Geometry check sheet. Reference: drawing and pictorial views, mm from the part's lowest x, y, z. Give positions to 0.01 mm unless a question says otherwise; leave off trailing zeros. Order: outer loops, then holes, each group sorted by start corner. A loop starts at its lowest first (then second) coordinate and runs counter-clockwise, first axis right, second up. Notation, with made-up numbers: M -28,58.25 L 8,58.25 A3 ccw 8,63.25 Z; hole C 36.5,78 d7. An arc over 180 degrees is marked long. Use CSV: the item, a comma, the result in double quotes. Start each with the question number.
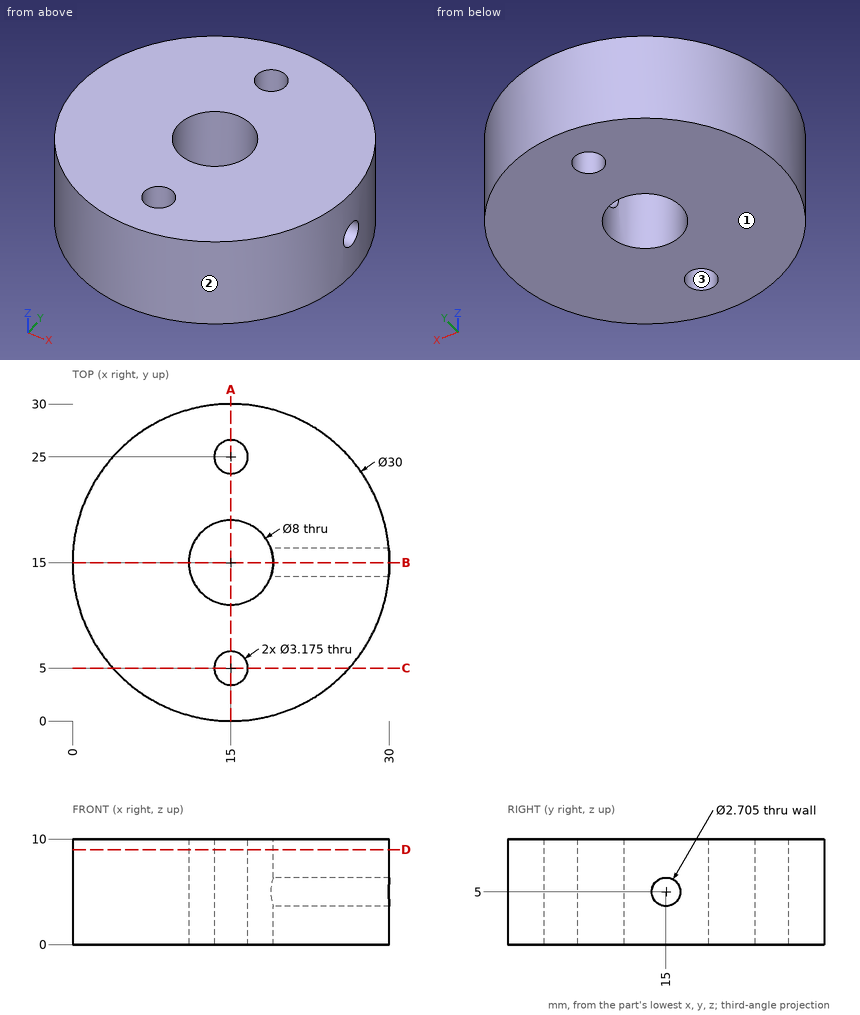
(1) Draft check along X on the marked faces 1, 2 and 3. Enter one of: +X half, -X half, draft (parallel to the pull), parting line (faces both ways), or undercut.
(2) Sectioned sample at B-B on y = 15. Record the cut outline in (x, z), then the cut area to 3 significant figures.
(3) Go/stop test with flat-tipped pins: P1, Ø5, axis at y = 24.5, z = 4.5, coming from the -X side; P2, Ø2, axis at y = 6, z = 5.5, coming from the +X side; P3, Ø7, axis at x = 15, y = 15, coming from the -Z side; P4, Ø3, axis at y = 23, z = 8.5, coming from the +X side. Record where each tip stops, or that it passes through.
(4) Sectioned sample at D-D on z = 9. Record the cut outline in (x, y) (1 decimal), then the cut area to 3 significant figures.
(5) Sectioned sample at C-C on y = 5. Record the cut outline in (x, z), then the cut area to 3 significant figures.
(6) Sectioned sample at A-A on x = 15. Record the cut outline in (y, z), then the cut area to 4 significant figures.
(7) Thickness scan on line 1 (Y direction, x = 15, z = 4.75); line 2 (X direction, y = 11.5, z = 4.5); line 3 (Y direction, x = 25.5, z = 1.5). Record the ranges inside material, lowest first.
Responses:
1,face 1,"draft"
1,face 2,"parting line"
1,face 3,"undercut"
2,outline,"M 0,0 L 11,0 L 11,10 L 0,10 Z; M 19,0 L 30,0 L 30,3.65 L 19,3.65 Z; M 19,6.35 L 30,6.35 L 30,10 L 19,10 Z"
2,area,"190 mm2"
3,P1,"x = 1.73"
3,P2,"x = 27.69"
3,P3,"through"
3,P4,"x = 28.52"
4,outline,"C 15,15 d30; hole C 15,15 d8; hole C 15,5 d3.2; hole C 15,25 d3.2"
4,area,"641 mm2"
5,outline,"M 3.82,0 L 13.41,0 L 13.41,10 L 3.82,10 Z; M 16.59,0 L 26.18,0 L 26.18,10 L 16.59,10 Z"
5,area,"192 mm2"
6,outline,"M 0,0 L 3.41,0 L 3.41,10 L 0,10 Z; M 6.59,0 L 11,0 L 11,10 L 6.59,10 Z; M 19,0 L 23.41,0 L 23.41,10 L 19,10 Z; M 26.59,0 L 30,0 L 30,10 L 26.59,10 Z"
6,area,"156.5 mm2"
7,line 1,"0 to 3.41, 6.59 to 11, 19 to 23.41, 26.59 to 30"
7,line 2,"0.41 to 13.06, 16.94 to 29.59"
7,line 3,"4.29 to 25.71"
